```python
from build123d import *

# Parameters (mm, degrees)
SKETCH002_R      = 9
EXTRUDE002_DEPTH = 2
SKETCH001_W      = 35
SKETCH001_H      = 40
EXTRUDE001_DEPTH = 6
SKETCH_R         = 2.5
EXTRUDE_DEPTH    = 8


with BuildPart() as extrude002:
    # Sketch002 (on Sketch) → Extrude002 (new body)
    with BuildSketch(Plane.XY):
        with Locations((-39, -12)):
            Circle(SKETCH002_R)
        with Locations((39, -12)):
            Circle(SKETCH002_R)
    extrude(amount=EXTRUDE002_DEPTH)


with BuildPart() as extrude_handle_notch:
    # Sketch001 → Extrude001 (new body)
    with BuildSketch(Plane.XY):
        with Locations((0, 20)):
            Rectangle(SKETCH001_W, SKETCH001_H)
    extrude(amount=EXTRUDE001_DEPTH)


with BuildPart() as cut001:
    # Sketch → Extrude (new body)
    with BuildSketch(Plane.XY):
        with BuildLine():
            Line((-50, 19), (-50, -19))
            Line((-50, -19), (-13.191508, -33.496031))
            ThreePointArc((-13.191508, -33.496031), (0, -36), (13.191508, -33.496031))
            Line((50, -19), (13.191508, -33.496031))
            Line((50, 19), (50, -19))
            Line((50, 19), (13.191508, 33.496031))
            ThreePointArc((13.191508, 33.496031), (0, 36), (-13.191508, 33.496031))
            Line((-50, 19), (-13.191508, 33.496031))
        make_face()
        with Locations((-42, 0)):
            Circle(SKETCH_R, mode=Mode.SUBTRACT)
        with Locations((42, 0)):
            Circle(SKETCH_R, mode=Mode.SUBTRACT)
        with Locations((-20, -15)):
            Circle(SKETCH_R, mode=Mode.SUBTRACT)
    extrude(amount=EXTRUDE_DEPTH)

    # Cut: cut Extrude Handle Notch
    add(extrude_handle_notch.part, mode=Mode.SUBTRACT)

    # Cut001: cut Extrude002
    add(extrude002.part, mode=Mode.SUBTRACT)


solid = cut001.part
```
Source: CAD feature listing. Evaluate the final solid. Frame: model axes, mm. A direction names the side the tool comes from. Round coordinates to 2 decimals unless told otherwise and drop trailing zeros. Loops run counter-clockwise (first coordinate to the right, second up) from the corner with the lowest first, then second, coordinate; pieces in that order, holes last. Notation, with made-up numbers: M -18,48.5 L 36,48.5 A21 cw 36,85.5 Z; hole C 79.5,50.5 d10. An arc over 180 degrees is marked long. Put each result on its own line as item: value.
(1) Pull-direction query (X, two-part tool) for faces 4 (the face through (0, -36, 4)), 5 (the face through (-31.85, 26.15, 3.94)), 6 (the face through (0, 0, 3)); classes: released by +X, released by -X, zero draft, split by the parting line, or undercut.
Solutions:
face 4: split by the parting line
face 5: released by -X
face 6: undercut
(2) First-contact query: pin 1 (3 mm diameter, centred on x = 2.5, z = 3, fed in from -Y); pin 2 (14.5 mm diameter, centred on x = -39, y = -12, fed in from -Z); pin 3 (4.5 mm diameter, centred on x = -20, y = -15, fed in from -Z); pin 4 (2 mm diameter, centred on x = 6, y = 6.5, fed in from -Z). Flat tips, straight axial feed; report the tip coordinate or a pass-through.
Solutions:
pin 1: y = -35.99
pin 2: z = 2
pin 3: through
pin 4: z = 6
(3) Section C-C, the plane x = -20. Return loops of the section in (y, z), and give its area (3 significant figures).
Solutions:
outline: M -30.81,0 L -17.5,0 L -17.5,8 L -30.81,8 Z; M -12.5,0 L 30.81,0 L 30.81,8 L -12.5,8 Z
area: 453 mm²
(4) Ray query, line 1 (X direction, y = 11.5, z = 1); line 2 (X direction, y = -14.5, z = 0.5); line 3 (Y direction, x = 39, z = 0.45). Return the intervals inside material, ascending. Write a range as [from, to].
Solutions:
line 1: [-50, -17.5], [17.5, 50]
line 2: [-50, -47.65], [-30.35, -22.45], [-17.55, 30.35], [47.65, 50]
line 3: [-23.33, -21], [-3, 23.33]
(5) Section A-A, the plane z = 4.5. Return loops of the section in (x, y).
Solutions:
outline: M -50,-19 L -13.19,-33.5 A36 ccw 13.19,-33.5 L 50,-19 L 50,19 L 17.5,31.8 L 17.5,0 L -17.5,0 L -17.5,31.8 L -50,19 Z; hole C -42,0 d5; hole C -20,-15 d5; hole C 42,0 d5
(6) Section D-D, the plane y = -1. Return loops of the section in (x, z).
Solutions:
outline: M -50,0 L -44.29,0 L -44.29,8 L -50,8 Z; M -39.71,0 L 39.71,0 L 39.71,8 L -39.71,8 Z; M 44.29,0 L 50,0 L 50,8 L 44.29,8 Z
(7) Access query for faces 1 (the face through (-17.5, 16, 3)), 2 (the face through (-22.5, -14.9, 3.9)), 3 (the face through (-46.14, -17.48, 0.99)). Directions: +Z, -Z, +X, -X, +Y, -Y. A direction counts if a zero-diameter tool reaches every point of the face in a straight line with its end or side. Return the directions, or none.
Solutions:
face 1: -Z, +Y
face 2: +Z, -Z
face 3: -Z
(8) Section B-B, the plane y = -15. Return loops of the section in (x, z).
Solutions:
outline: M -50,0 L -47.49,0 L -47.49,2 L -30.51,2 L -30.51,0 L -22.5,0 L -22.5,8 L -50,8 Z; M -17.5,0 L 30.51,0 L 30.51,2 L 47.49,2 L 47.49,0 L 50,0 L 50,8 L -17.5,8 Z
